from build123d import *

# Parameters (mm, degrees)
SKETCH1_R           = 2
BOSS_EXTRUDE1_DEPTH = 8


with BuildPart() as part:
    # Sketch1 → Boss-Extrude1 (new body)
    with BuildSketch(Plane(origin=(0, 0, 0), x_dir=(1, 0, 0), z_dir=(0, 1, 0))):
        with BuildLine():
            Line((-125.897027312, 145.777430233), (-117.648504662, 124.298055814))
            ThreePointArc((-117.648504662, 124.298055814), (-113.242326544, 118.710021986), (-106.446126512, 116.6))
            Line((-106.446126512, 116.6), (106.446126512, 116.6))
            ThreePointArc((106.446126512, 116.6), (113.242326544, 118.710021986), (117.648504662, 124.298055814))
            Line((117.648504662, 124.298055814), (125.897027312, 145.777430233))
            ThreePointArc((125.897027312, 145.777430233), (145.277430233, 154.402972688), (153.902972688, 135.022569767))
            Line((153.902972688, 135.022569767), (139.002972688, 96.222569767))
            ThreePointArc((139.002972688, 96.222569767), (133.495250041, 89.237527482), (125, 86.6))
            Line((125, 86.6), (-125, 86.6))
            ThreePointArc((-125, 86.6), (-133.495250041, 89.237527482), (-139.002972688, 96.222569767))
            Line((-139.002972688, 96.222569767), (-153.902972688, 135.022569767))
            ThreePointArc((-153.902972688, 135.022569767), (-145.277430233, 154.402972688), (-125.897027312, 145.777430233))
        make_face()
        with Locations(Location((-125, 101.6, 0), (0, 0, 270))):
            Circle(SKETCH1_R, mode=Mode.SUBTRACT)
        with Locations(Location((125, 101.6, 0), (0, 0, 270))):
            Circle(SKETCH1_R, mode=Mode.SUBTRACT)
        with BuildLine():
            Line((-145.4, 143.65), (-134.4, 143.65))
            ThreePointArc((-134.4, 143.65), (-131.15, 140.4), (-134.4, 137.15))
            Line((-134.4, 137.15), (-145.4, 137.15))
            ThreePointArc((-145.4, 137.15), (-148.65, 140.4), (-145.4, 143.65))
        make_face(mode=Mode.SUBTRACT)
        with BuildLine():
            Line((145.4, 137.15), (134.4, 137.15))
            ThreePointArc((134.4, 137.15), (131.15, 140.4), (134.4, 143.65))
            Line((134.4, 143.65), (145.4, 143.65))
            ThreePointArc((145.4, 143.65), (148.65, 140.4), (145.4, 137.15))
        make_face(mode=Mode.SUBTRACT)
    extrude(amount=BOSS_EXTRUDE1_DEPTH)


solid = part.part
Could you check a few things on this model? Use its own coordinates, in mm. A direction names the side the tool comes from. Round coordinates to 2 decimals unless told otherwise and drop trailing zeros. Order: outer loops, then holes, each group sorted by start corner. A loop starts at its lowest first (then second) coordinate and runs counter-clockwise, first axis right, second up.
Q1. Imagine slicing it at C-C, the plane x = -54.5. List the corners of the cut face in (y, z) for me, then the cut area to 3 significant figures.
Geometry says:
outline: (0, -116.6) - (8, -116.6) - (8, -86.6) - (0, -86.6) - close
area: 240 mm2
Q2. Thinking about a two-plate mould opening in X: for faces 1 (the face through (133.6, 3.94, -89.31)), 2 (the face through (148.65, 3.94, -140.47)), 3 (the face through (2, 8, -114)), which applies, released by +X, released by -X, zero draft, split by the parting line, or undercut?
Geometry says:
face 1: released by +X
face 2: undercut
face 3: zero draft
Q3. Which directions (+Z, -Z, +X, -X, +Y, -Y) give clear straight access to the entire face, cutting with the end or side of a thin tool? Please do faces 4 (the face through (140, 4, -137.15)), 5 (the face through (2, 0, -114)), 6 (the face through (-1, 4, -116.6)).
Geometry says:
face 4: +Y, -Y
face 5: +Z, -Z, +X, -X, -Y
face 6: -Z, +Y, -Y
Q4. Imagine slicing it at D-D, the plane z = -108. List the corners of the cut face in (x, y) for me.
Geometry says:
outline: (-143.53, 0) - (143.53, 0) - (143.53, 8) - (-143.53, 8) - close
Q5. I'm going to push flat-ended pins straight in: P1, Ø4, axis at x = -140, y = 4.5, coming from the +Z side; P2, Ø3, axis at x = 6, z = -96, coming from the -Y side; P3, Ø2.5, axis at x = -141.5, y = 5.5, coming from the -Z side; P4, Ø2.5, axis at x = 5, y = 5.5, coming from the -Z side. Where does each tip first touch, or does it pass through?
Geometry says:
P1: stops at z = -94.12
P2: stops at y = 0
P3: stops at z = -155.4
P4: stops at z = -116.6
Q6. Imagine slicing it at B-B, the plane z = -150. List the corners of the cut face in (x, y) for me.
Geometry says:
outline: (-151.43, 0) - (-128.37, 0) - (-128.37, 8) - (-151.43, 8) - close; (128.37, 0) - (151.43, 0) - (151.43, 8) - (128.37, 8) - close
Q7. Imagine slicing it at A-A, the plane y = 1.75. List the corners of the cut face in (x, z) for me, then the cut area to 3 significant figures.
Geometry says:
outline: (-153.9, -135.02) arc R15 ccw to (-125.9, -145.78) - (-117.65, -124.3) arc R12 cw to (-106.45, -116.6) - (106.45, -116.6) arc R12 cw to (117.65, -124.3) - (125.9, -145.78) arc R15 ccw to (153.9, -135.02) - (139, -96.22) arc R15 ccw to (125, -86.6) - (-125, -86.6) arc R15 ccw to (-139, -96.22) - close; hole (-145.4, -143.65) - (-134.4, -143.65) arc R3.25 ccw to (-134.4, -137.15) - (-145.4, -137.15) arc R3.25 ccw to start; hole circle Ø4 at (-125, -101.6); hole circle Ø4 at (125, -101.6); hole (134.4, -143.65) - (145.4, -143.65) arc R3.25 ccw to (145.4, -137.15) - (134.4, -137.15) arc R3.25 ccw to start
area: 10,500 mm2
Q8. Please list where these lines run through material, in increasing order: probe 1 along X at (y, z) = (5.5, -101.6); probe 2 along X at (y, z) = (5.75, -141); probe 3 along X at (y, z) = (5, -138).
Geometry says:
probe 1: x = -141.07 to -127, -123 to 123, 127 to 141.07
probe 2: x = -154.89 to -148.59, -131.21 to -124.06, 124.06 to 131.21, 148.59 to 154.89
probe 3: x = -154.71 to -147.59, -132.21 to -122.91, 122.91 to 132.21, 147.59 to 154.71
